Build history of the part. All positions in model axes, mm. A direction names the side the tool comes from. Round coordinates to 2 decimals unless told otherwise and drop trailing zeros. Loops run counter-clockwise (first coordinate to the right, second up) from the corner with the lowest first, then second, coordinate; pieces in that order, holes last. Notation, with made-up numbers: (22.25, 24.5) - (27.25, 24.5) arc R12 cw to (27.25, 45.5) - close; hole circle Ø8 at (55, 20). An arc over 180 degrees is marked (long way). Use one line per item in the form item = value. Start each with the question number.
Q1. Saw through at A-A (y = 2). Give the cut face in (x, z), then the cut area to 3 significant figures.
Q2. 3-axis set-ups, long thin cutter, end or side, ignore diameter. For faces 4 (the face through (-19.137, -4.781, -13.922)), 5 (the face through (0, -4.5, -18)), 6 (the face through (-16.9, 16.269, 10.484)), 7 (the face through (22, 13, 11.536)), 8 (the face through (-0.1, 31.5, 18.2)): which of +Z, -Z, +X, -X, +Y, -Y reach the whole face in a straight line?
Q3. Pin check, flat tips, straight feed: pin 1 (1.5 mm diameter, centred on y = 22.5, z = 3.5, fed in from -X); pin 2 (2 mm diameter, centred on x = 24.5, y = 12, fed in from +Z); pin 3 (8 mm diameter, centred on y = 9, z = 8.5, fed in from +X). Stop position of each tip, or through.
Q4. Saw through at D-D (y = 17.5). Count the separate pieces of the cut face and the enclosed holes in it, then the cut area to 3 significant figures.
Q5. Saw through at B-B (x = -8). Give the cut face in (y, z).
Q6. Drill centre lines: line 1 (X direction, y = -3.45, z = 0); line 2 (Y direction, x = 8, z = -9.5); line 3 (X direction, y = 21.5, z = 5). Where is each one in solid material? Low to high.
Q7. Mould opens along Y. For faces 1 (the face through (-16.954, 16.269, -10.538)), 2 (the face through (0, 33, 0)), 3 (the face through (15, 11, 0)) say: released by +Y, released by -Y, zero draft, split by the parting line, or undercut.
Q8. Saw through at C-C (x = 0). Give the cut face in (y, z), then the cut area to 3 significant figures.
```python
from build123d import *

# Parameters (mm, degrees)
SKETCH1_W                       = 30
SKETCH1_H                       = 30
BOSS_EXTRUDE1_DEPTH             = 28.5
CUT_EXTRUDE1_DEPTH              = 53.091266063
CUT_EXTRUDE1_DEPTH_BACK         = 53.091266063
SKETCH3_R                       = 2.15
SKETCH3_R_2                     = 1.6
CUT_EXTRUDE2_DEPTH              = 53.091266063
CUT_EXTRUDE3_DEPTH              = 53.091266063
CUT_EXTRUDE3_DEPTH_BACK         = 53.091266063
SKETCH5_OUTSIDE_W               = 76.998
SKETCH5_OUTSIDE_H               = 76.998
SKETCH5_OUTSIDE_R               = 28.5
CUT_EXTRUDE4_DEPTH              = 53.091266063
CUT_EXTRUDE4_DEPTH_BACK         = 53.091266063
SKETCH7_R                       = 5
CUT_EXTRUDE5_DEPTH              = 4.5
SKETCH3_3_R                     = 1.6
CUT_EXTRUDE6_DEPTH              = 50.406816501
SKETCH8_R                       = 5
CUT_EXTRUDE7_DEPTH              = 4.5
SKETCH9_W                       = 0.901470183
SKETCH9_H                       = 10
BOSS_EXTRUDE2_DEPTH             = 33.5
CUT_EXTRUDE9_DEPTH              = 50.406816501
CUT_EXTRUDE9_DEPTH_BACK         = 50.406816501
SKETCH10_R                      = 3.2
CUT_EXTRUDE10_REACH             = 56.333
SKETCH11_R                      = 3.2
CUT_EXTRUDE10_DIRECTION_2_DEPTH = 55.33261927


with BuildPart() as part:
    # Sketch1 → Boss-Extrude1 (new, symmetric)
    with BuildSketch(Plane.XY):
        Polygon((-28.5, 0), (-20, 33), (20, 33), (28.5, 0), (28.5, -7), (-28.5, -7), align=None)
        with Locations((0, 15)):
            Rectangle(SKETCH1_W, SKETCH1_H, mode=Mode.SUBTRACT)
    extrude(amount=BOSS_EXTRUDE1_DEPTH, both=True)

    # Sketch3 → Cut-Extrude1 (cut, two sides: drawn at the far end of the back side and taken through both)
    with BuildSketch(Plane(origin=(0, 0, 0), x_dir=(1, 0, 0), z_dir=(0, 1, 0)).offset(-CUT_EXTRUDE1_DEPTH_BACK)):
        with Locations(Location((-19.401470183, 8.03635208, 0), (0, 0, 270))):
            Circle(SKETCH3_R)
        with Locations(Location((-20, 0, 0), (0, 0, 270))):
            Circle(SKETCH3_R_2)
        with Locations(Location((19.401470183, 8.03635208, 0), (0, 0, 270))):
            Circle(SKETCH3_R)
        with Locations(Location((20, 0, 0), (0, 0, 270))):
            Circle(SKETCH3_R_2)
        with Locations(Location((19.401470183, -8.03635208, 0), (0, 0, 270))):
            Circle(SKETCH3_R)
        with Locations(Location((-19.401470183, -8.03635208, 0), (0, 0, 270))):
            Circle(SKETCH3_R)
    extrude(amount=CUT_EXTRUDE1_DEPTH + CUT_EXTRUDE1_DEPTH_BACK, mode=Mode.SUBTRACT)

    # Sketch4 → Cut-Extrude2 (cut, through all)
    with BuildSketch(Plane(origin=(0, 0, 0), x_dir=(1, 0, 0), z_dir=(0, 1, 0))):
        with BuildLine():
            Line((28.5, 11.53635208), (19.401470183, 11.53635208))
            ThreePointArc((19.401470183, 11.53635208), (16.926596449, 10.511225814), (15.901470183, 8.03635208))
            Line((15.901470183, 8.03635208), (15.901470183, 5))
            Line((15.901470183, 5), (15, 5))
            Line((15, 5), (15, -5))
            Line((15, -5), (15.901470183, -5))
            Line((15.901470183, -5), (15.901470183, -8.03635208))
            ThreePointArc((15.901470183, -8.03635208), (16.926596449, -10.511225814), (19.401470183, -11.53635208))
            Line((19.401470183, -11.53635208), (28.5, -11.53635208))
            Line((28.5, -11.53635208), (28.5, 11.53635208))
        make_face()
        with BuildLine():
            Line((-15.901470183, -5), (-15.901470183, -8.03635208))
            ThreePointArc((-15.901470183, -8.03635208), (-16.926596449, -10.511225814), (-19.401470183, -11.53635208))
            Line((-19.401470183, -11.53635208), (-28.5, -11.53635208))
            Line((-28.5, -11.53635208), (-28.5, 11.53635208))
            Line((-28.5, 11.53635208), (-19.401470183, 11.53635208))
            ThreePointArc((-19.401470183, 11.53635208), (-16.926596449, 10.511225814), (-15.901470183, 8.03635208))
            Line((-15.901470183, 8.03635208), (-15.901470183, 5))
            Line((-15.901470183, 5), (-15, 5))
            Line((-15, 5), (-15, -5))
            Line((-15, -5), (-15.901470183, -5))
        make_face()
    extrude(amount=CUT_EXTRUDE2_DEPTH, mode=Mode.SUBTRACT)

    # Sketch5 outside → Cut-Extrude3 (cut, two sides: drawn at the far end of the back side and taken through both)
    with BuildSketch(Plane(origin=(0, 0, 0), x_dir=(1, 0, 0), z_dir=(0, 1, 0)).offset(-CUT_EXTRUDE3_DEPTH_BACK)):
        Rectangle(SKETCH5_OUTSIDE_W, SKETCH5_OUTSIDE_H)
        with Locations(Location((0, 0, 0), (0, 0, 270))):
            Circle(SKETCH5_OUTSIDE_R, mode=Mode.SUBTRACT)
    extrude(amount=CUT_EXTRUDE3_DEPTH + CUT_EXTRUDE3_DEPTH_BACK, mode=Mode.SUBTRACT)

    # Sketch6 → Cut-Extrude4 (cut, two sides: drawn at the far end of the back side and taken through both)
    with BuildSketch(Plane(origin=(0, 0, 0), x_dir=(1, 0, 0), z_dir=(0, 1, 0)).offset(-CUT_EXTRUDE4_DEPTH_BACK)):
        with BuildLine():
            Line((-16.506558795, -23.233241632), (16.506558795, -23.233241632))
            ThreePointArc((16.506558795, -23.233241632), (0, -28.5), (-16.506558795, -23.233241632))
        make_face()
        with BuildLine():
            Line((-16.506558795, 23.233241632), (16.506558795, 23.233241632))
            ThreePointArc((16.506558795, 23.233241632), (0, 28.5), (-16.506558795, 23.233241632))
        make_face()
    extrude(amount=CUT_EXTRUDE4_DEPTH + CUT_EXTRUDE4_DEPTH_BACK, mode=Mode.SUBTRACT)

    # Sketch7 → Cut-Extrude5 (cut)
    with BuildSketch(Plane.XZ.offset(7)):
        with Locations((-14.142135624, 14.142135624)):
            Circle(SKETCH7_R)
        with Locations(Location((14.142135624, -14.142135624, 0), (0, 0, 180))):
            Circle(SKETCH7_R)
        with Locations((-14.142135624, -14.142135624)):
            Circle(SKETCH7_R)
        with Locations((14.142135624, 14.142135624)):
            Circle(SKETCH7_R)
    extrude(amount=-CUT_EXTRUDE5_DEPTH, mode=Mode.SUBTRACT)

    # Sketch3<3> → Cut-Extrude6 (cut, through all)
    with BuildSketch(Plane(origin=(0, 0, 0), x_dir=(1, 0, 0), z_dir=(0, 1, 0))):
        with Locations(Location((0, 20, 0), (0, 0, 270))):
            Circle(SKETCH3_3_R)
        with Locations(Location((0, -20, 0), (0, 0, 270))):
            Circle(SKETCH3_3_R)
    extrude(amount=-CUT_EXTRUDE6_DEPTH, mode=Mode.SUBTRACT)

    # Sketch8 → Cut-Extrude7 (cut)
    with BuildSketch(Plane(origin=(0, 0, 0), x_dir=(1, 0, 0), z_dir=(0, 1, 0))):
        with Locations((0, -20)):
            Circle(SKETCH8_R)
        with Locations((0, 20)):
            Circle(SKETCH8_R)
        with Locations(Location((-20, 0, 0), (0, 0, 270))):
            Circle(SKETCH8_R)
        with Locations(Location((20, 0, 0), (0, 0, 270))):
            Circle(SKETCH8_R)
    extrude(amount=-CUT_EXTRUDE7_DEPTH, mode=Mode.SUBTRACT)

    # Sketch9 → Boss-Extrude2 (add)
    with BuildSketch(Plane(origin=(0, 33, 0), x_dir=(1, 0, 0), z_dir=(0, 1, 0))):
        with Locations((-15.450735092, 0)):
            Rectangle(SKETCH9_W, SKETCH9_H)
        with Locations((15.450735092, 0)):
            Rectangle(SKETCH9_W, SKETCH9_H)
    extrude(amount=-BOSS_EXTRUDE2_DEPTH)

    # Sketch10 → Cut-Extrude9 (cut, two sides: drawn at the far end of the back side and taken through both)
    with BuildSketch(Plane(origin=(0, 0, 0), x_dir=(0, 0, -1), z_dir=(1, 0, 0)).offset(-CUT_EXTRUDE9_DEPTH_BACK)):
        with Locations((0, 15)):
            Circle(SKETCH10_R)
    extrude(amount=CUT_EXTRUDE9_DEPTH + CUT_EXTRUDE9_DEPTH_BACK, mode=Mode.SUBTRACT)

    # Sketch11 → Cut-Extrude10 (cut, up to next)
    with BuildSketch(Plane(origin=(0, 33, 0), x_dir=(1, 0, 0), z_dir=(0, 1, 0)), mode=Mode.PRIVATE) as cut_extrude10_sk1:
        with Locations(Location((0, 15, 0), (0, 0, 90))):
            Circle(SKETCH11_R)
    cut_extrude10_tool1 = extrude(cut_extrude10_sk1.sketch, amount=-CUT_EXTRUDE10_REACH, mode=Mode.PRIVATE) & part.part
    # Sketch11 → Cut-Extrude10 (cut, up to next)
    with BuildSketch(Plane(origin=(0, 33, 0), x_dir=(1, 0, 0), z_dir=(0, 1, 0)), mode=Mode.PRIVATE) as cut_extrude10_sk2:
        with Locations(Location((0, -15, 0), (0, 0, 90))):
            Circle(SKETCH11_R)
    cut_extrude10_tool2 = extrude(cut_extrude10_sk2.sketch, amount=-CUT_EXTRUDE10_REACH, mode=Mode.PRIVATE) & part.part
    add(cut_extrude10_tool1.solids().sort_by_distance((0, 33, -15))[0], mode=Mode.SUBTRACT)
    add(cut_extrude10_tool2.solids().sort_by_distance((0, 33, 15))[0], mode=Mode.SUBTRACT)

    # Sketch11 → Cut-Extrude10 direction 2 (cut)
    with BuildSketch(Plane(origin=(0, 33, 0), x_dir=(1, 0, 0), z_dir=(0, 1, 0))):
        with Locations(Location((0, 15, 0), (0, 0, 90))):
            Circle(SKETCH11_R)
        with Locations(Location((0, -15, 0), (0, 0, 90))):
            Circle(SKETCH11_R)
    extrude(amount=CUT_EXTRUDE10_DIRECTION_2_DEPTH, mode=Mode.SUBTRACT)


solid = part.part
```
Report:
q1.outline = (-26.06, -11.54) arc R28.5 ccw to (-16.51, -23.23) - (-15, -23.23) - (-15, 23.23) - (-16.51, 23.23) arc R28.5 ccw to (-26.06, 11.54) - (-19.4, 11.54) arc R3.5 cw to (-15.9, 8.04) - (-15.9, -8.04) arc R3.5 cw to (-19.4, -11.54) - close; (15, -23.23) - (16.51, -23.23) arc R28.5 ccw to (26.06, -11.54) - (19.4, -11.54) arc R3.5 cw to (15.9, -8.04) - (15.9, 8.04) arc R3.5 cw to (19.4, 11.54) - (26.06, 11.54) arc R28.5 ccw to (16.51, 23.23) - (15, 23.23) - close
q1.area = 387 mm²
q2.face_4 = -Y
q2.face_5 = none
q2.face_6 = -X, +Y
q2.face_7 = +X, +Y
q2.face_8 = +Y
q3.pin_1 = -15.9
q3.pin_2 = 16.12
q3.pin_3 = 26.06
q4.separate_pieces = 4
q4.enclosed_holes = 0
q4.area = 363 mm²
q5.outline = (-7, -23.23) - (0, -23.23) - (0, 23.23) - (-7, 23.23) - close; (30, -23.23) - (33, -23.23) - (33, 23.23) - (30, 23.23) - close
q6.line_1 = -28.5 to -25, -15 to 15, 25 to 28.5
q6.line_2 = -7 to 0, 30 to 33
q6.line_3 = -15.9 to -15, 15 to 15.9
q7.face_1 = zero draft
q7.face_2 = released by +Y
q7.face_3 = undercut
q8.outline = (-7, -23.23) - (-4.5, -23.23) - (-4.5, -21.6) - (-7, -21.6) - close; (-7, -18.4) - (-4.5, -18.4) - (-4.5, -15) - (0, -15) - (0, 15) - (-4.5, 15) - (-4.5, 18.4) - (-7, 18.4) - close; (-7, 21.6) - (-4.5, 21.6) - (-4.5, 23.23) - (-7, 23.23) - close; (30, -23.23) - (33, -23.23) - (33, -18.2) - (30, -18.2) - close; (30, -11.8) - (33, -11.8) - (33, 11.8) - (30, 11.8) - close; (30, 18.2) - (33, 18.2) - (33, 23.23) - (30, 23.23) - close
q8.area = 336 mm²
